Geometry check sheet. Reference: drawing and pictorial views, mm from the part's lowest x, y, z. A direction names the side the tool comes from. Give positions to 0.01 mm unless a question says otherwise; leave off trailing zeros. Loops run counter-clockwise (first coordinate to the right, second up) from the corner with the lowest first, then second, coordinate; pieces in that order, holes last. Notation, with made-up numbers: (-9, 0.25) - (22, 0.25) arc R19 cw to (22, 30.25) - close; hole circle Ø5 at (43.5, 50). An arc over 180 degrees is marked (long way). One line per question, with ' | ' between items. Start each with the question number.
1. Section check D-D, the plane z = 1.5. Enter the section's corners in (x, y), then the cut area to 3 significant figures.
2. Section check B-B, the plane z = 5. Enter the section's corners in (x, y).
3. Section check A-A, the plane x = 21. Enter the section's corners in (y, z), then the cut area to 3 significant figures.
4. Tool access check on the marked faces 4 and 5. Record the directions out of +Z, -Z, +X, -X, +Y, -Y that give a thin tool (end or side, any length) a straight path to the whole face; none if there is none.
5. Thickness scan on line 1 along Z through (x, y) = (21, 2.35); line 2 along X through (y, z) = (8.5, 8.5). Record the ranges inside material, lowest first. Write a range as from..to.
6. Mould release check, pull along Z, two halves, no side actions. Record for the marked faces 1, 2 and 3: +Z half, -Z half, draft (parallel to the pull), parting line (faces both ways), or undercut.
7. Depth check by flat-ended pin: pin 1 Ø5 at (y, z) = (18.5, 4.5) entering from +X; pin 2 Ø3 at (x, z) = (21.5, 7.5) entering from +Y. Enter the tip coordinate at first touch or a pass-through.
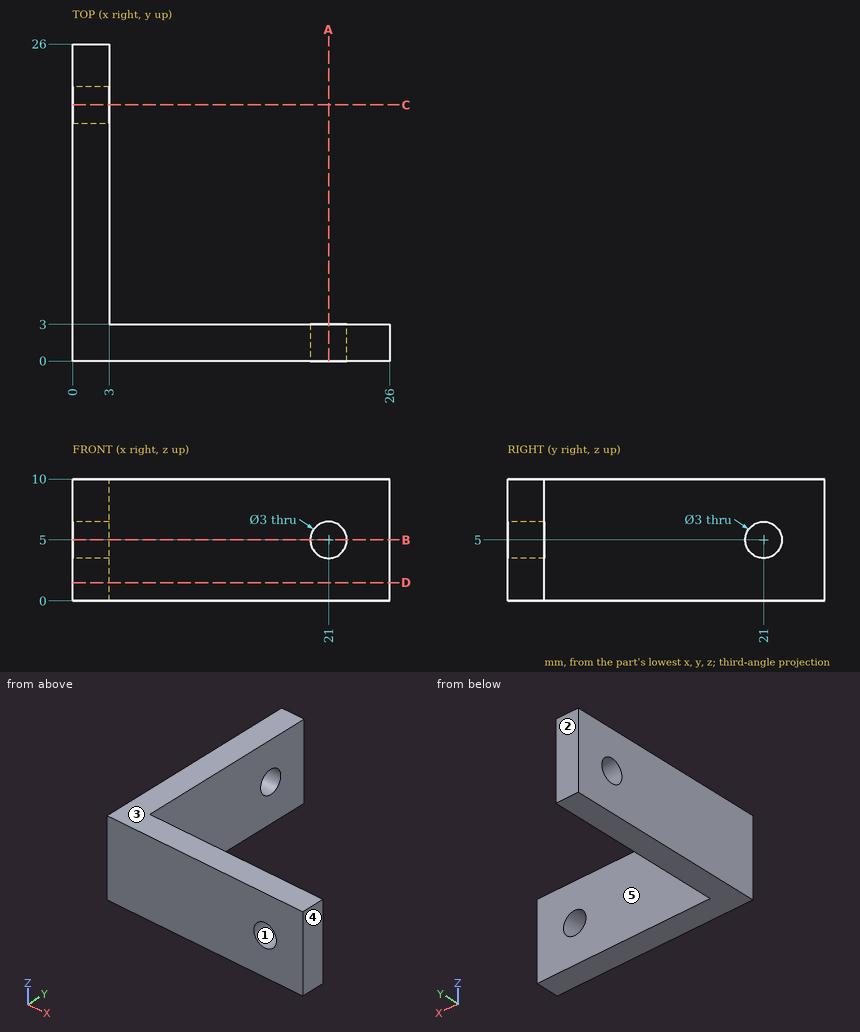
Results list:
1) outline: (0, 0) - (26, 0) - (26, 3) - (3, 3) - (3, 26) - (0, 26) - close | area: 147 mm²
2) outline: (0, 0) - (19.5, 0) - (19.5, 3) - (3, 3) - (3, 19.5) - (0, 19.5) - close; (0, 22.5) - (3, 22.5) - (3, 26) - (0, 26) - close; (22.5, 0) - (26, 0) - (26, 3) - (22.5, 3) - close
3) outline: (0, 0) - (3, 0) - (3, 3.5) - (0, 3.5) - close; (0, 6.5) - (3, 6.5) - (3, 10) - (0, 10) - close | area: 21.0 mm²
4) face 4: +Z, -Z, +X, +Y, -Y | face 5: +Z, -Z, +X, +Y
5) line 1: 0..3.5, 6.5..10 | line 2: 0..3
6) face 1: undercut | face 2: draft | face 3: +Z half
7) pin 1: x = 3 | pin 2: y = 3
